Check sheet for the drawn part. Datum: minimum x, y, z corner. Units: mm. A direction names the side the tool comes from. Give positions to 0.01 mm unless a question says otherwise; leave off trailing zeros. Order: outer loops, then holes, each group sorted by start corner. A loop starts at its lowest first (then second) coordinate and runs counter-clockwise, first axis right, second up.
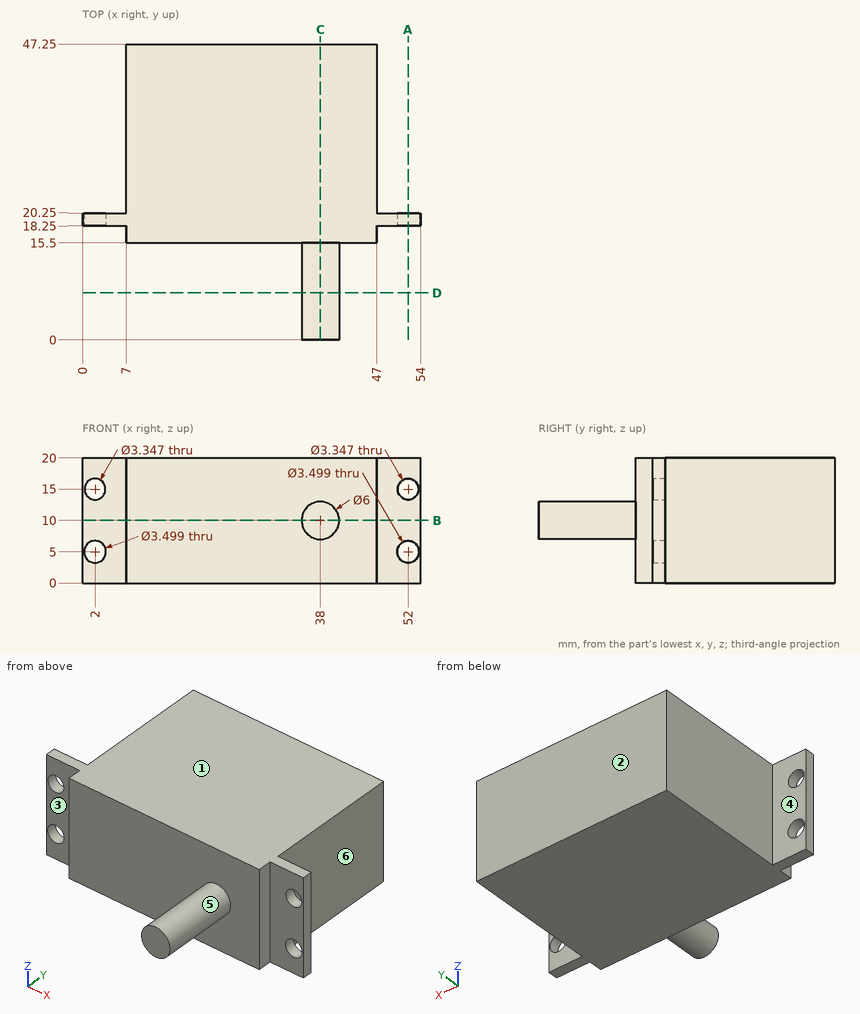
(1) Section check B-B, the plane z = 10. Enter the section's corners in (x, y), then the cut area to 3 significant figures.
Solved:
outline: (0, 18.25) - (7, 18.25) - (7, 15.5) - (35, 15.5) - (35, 0) - (41, 0) - (41, 15.5) - (47, 15.5) - (47, 18.25) - (54, 18.25) - (54, 20.25) - (47, 20.25) - (47, 47.25) - (7, 47.25) - (7, 20.25) - (0, 20.25) - close
area: 1,390 mm2
(2) Go/stop test with flat-tipped pins: pin 1 (3.5 mm diameter, centred on x = 51, z = 8, fed in from +Y); pin 2 (3 mm diameter, centred on x = 52, z = 15, fed in from +Y); pin 3 (10 mm diameter, centred on y = 27, z = 14.5, fed in from -X); pin 4 (3.5 mm diameter, centred on x = 50, z = 14, fed in from -Y). Record where each tip stops, or that it passes through.
Solved:
pin 1: stops at y = 20.25
pin 2: passes through
pin 3: stops at x = 7
pin 4: stops at y = 18.25
(3) Set-up check for the marked faces 4, 5 and 6: record each of +Z, -Z, +X, -X, +Y, -Y from which the full face is reachable in a straight line by a thin tool's end or side.
Solved:
face 4: +Z, -Z, -X, +Y
face 5: -Y
face 6: +Z, -Z, +X, +Y
(4) Section check C-C, the plane x = 38. Enter the section's corners in (y, z).
Solved:
outline: (0, 7) - (15.5, 7) - (15.5, 0) - (47.25, 0) - (47.25, 20) - (15.5, 20) - (15.5, 13) - (0, 13) - close
(5) Scan lines: line 1 (X direction, y = 19.3, z = 15); line 2 (Z direction, x = 52, y = 19); line 3 (Y direction, x = 11, z = 6.75). Record each from-to range of solid material in increasing order.
Solved:
line 1: x = 0 to 0.33, 3.67 to 50.33, 53.67 to 54
line 2: z = 0 to 3.25, 6.75 to 13.33, 16.67 to 20
line 3: y = 15.5 to 47.25
(6) Section check A-A, the plane x = 52. Enter the section's corners in (y, z), then the cut area to 3 significant figures.
Solved:
outline: (18.25, 0) - (20.25, 0) - (20.25, 3.25) - (18.25, 3.25) - close; (18.25, 6.75) - (20.25, 6.75) - (20.25, 13.33) - (18.25, 13.33) - close; (18.25, 16.67) - (20.25, 16.67) - (20.25, 20) - (18.25, 20) - close
area: 26.3 mm2
(7) Release check for a two-part mould opening along Y. For the marked faces 1, 2 and 3 record: pulls with the +Y half, pulls with the -Y half, needs draft (parallel to the pull), parting line crosses it, or undercut.
Solved:
face 1: needs draft
face 2: pulls with the +Y half
face 3: pulls with the -Y half
(8) Section check D-D, the plane y = 7.5. Enter the section's corners in (x, z), then the cut area to 3 significant figures.
Solved:
outline: circle Ø6 at (38, 10)
area: 28.3 mm2
